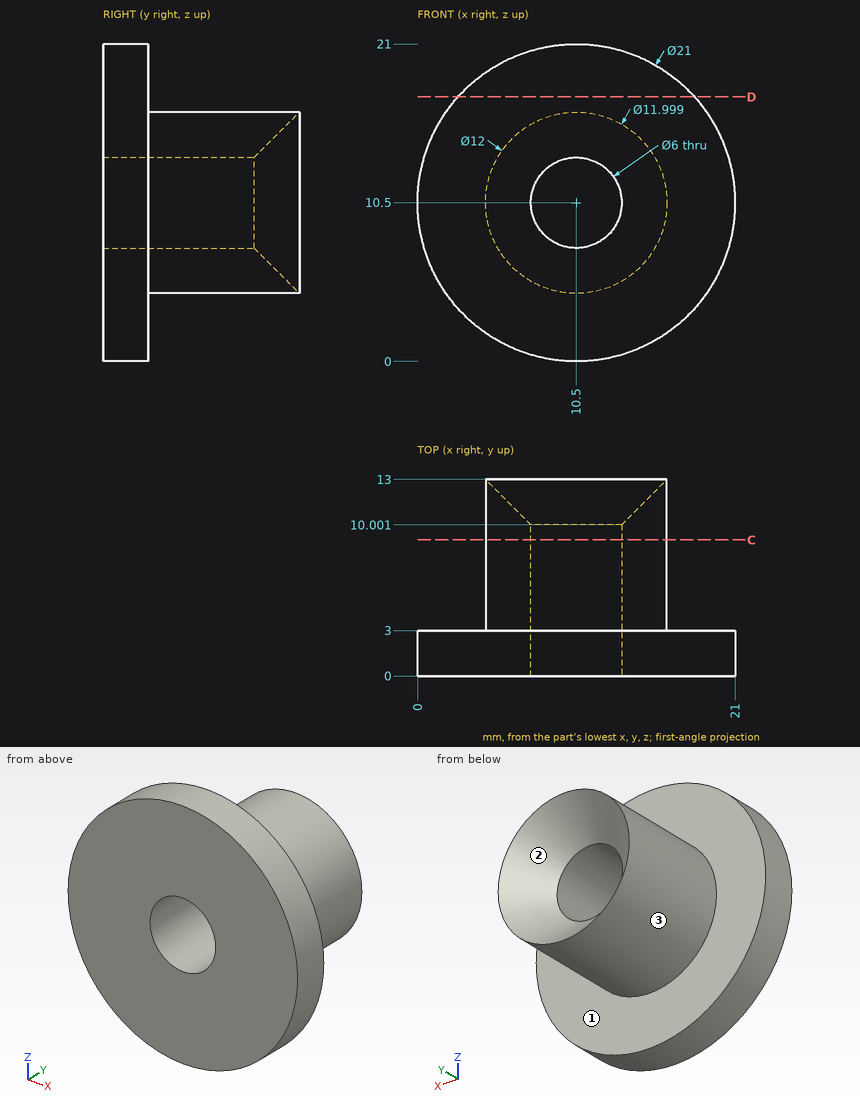
Source: three-view drawing plus pictorial views. Frame: mm from the lowest corner of the part. Round coordinates to 2 decimals unless told otherwise and drop trailing zeros. Loops run counter-clockwise (first coordinate to the right, second up) from the corner with the lowest first, then second, coordinate; pieces in that order, holes last.
1. Section query D-D on z = 17.5. Output: boundary loops of the cut face in (x, y).
2. Section query C-C on y = 9. Output: boundary loops of the cut face in (x, z).
3. Ray query, L1, parallel to X at y = 4.75, z = 10.5; L2, parallel to Z at x = 10.5, y = 2.5. Return the intervals inside material, ascending.
4. Mould query, pull axis Z, two halves, no side actions, for the marked faces 1, 2 and 3. Classes: released by +Z, released by -Z, zero draft, split by the parting line, or undercut.
5. Contact query for flat-ended pins moving along their axis: pin 1 (3.5 mm diameter, centred on x = 10.5, z = 10.5, fed in from -Y) (3 decimals); pin 2 (5 mm diameter, centred on y = 11, z = 12.5, fed in from +X); pin 3 (2 mm diameter, centred on y = 2.5, z = 12, fed in from -X); pin 4 (5 mm diameter, centred on y = 11, z = 16.5, fed in from +X) (1 decimal). Output: stop coordinate, or through.
Answers below:
1. outline: (2.67, 0) - (18.33, 0) - (18.33, 3) - (2.67, 3) - close
2. outline: circle Ø12 at (10.5, 10.5); hole circle Ø6 at (10.5, 10.5)
3. L1: x = 4.5 to 7.5, 13.5 to 16.5
3. L2: z = 0 to 7.5, 13.5 to 21
4. face 1: zero draft
4. face 2: undercut
4. face 3: split by the parting line
5. pin 1: passes through
5. pin 2: stops at x = 16.5
5. pin 3: stops at x = 0.01
5. pin 4: stops at x = 15.4
